Could you check a few things on this model? Use its own coordinates, in mm. A direction names the side the tool comes from. Coordinates: 2 decimals unless noted, no trailing zeros. Write each loop counter-clockwise with the first axis right and the second up, starting at its lowest first coordinate (ties: lowest second). Pieces come first, ordered by that corner, then holes.
Item 1: Which directions (+Z, -Z, +X, -X, +Y, -Y) give clear straight access to the entire face, cutting with the end or side of a thin tool? Please do faces 1 (the flat face through (-2, 2, -8.8)), 2 (the flat face through (-8.745, -7, 5)), 3 (the flat face through (-7.245, -5, 6)).
Item 2: I want a section at C-C on x = -13.5. Please give me the cut outline in (y, z), then the cut area to 3 significant figures.
Item 3: I want a section at B-B on y = -8. Please give me the cut outline in (x, z).
Item 4: If I drill on probe 1 along Z at (x, y) = (-4, -1.75); probe 2 along X at (y, z) = (-1.25, 0.5); probe 3 along Z at (x, y) = (-12.5, -1), over which ranges is the centre line in solid material (lowest first)?
Item 5: Thinking about a two-plate mould opening in X: for faces 4 (the flat face through (3.255, -3, 5)), 5 (the flat face through (1, 4, -19.7)), 6 (the flat face through (-8, -3, 8.8)), 7 (the cylindrical face through (1.54, 10.22, -5.87)), which applies, +X half, -X half, draft (parallel to the pull), parting line (faces both ways), or undercut?
Item 6: For P1, Ø1.6, axis at x = -3, y = -5.5, coming from the +Z side; P2, Ø1.5, axis at y = -3.5, z = 7, coming from the -X side; P3, Ø0.6, axis at y = 4, z = -20, coming from the -X side, each with a flat end and sliding along its axis, tell me the tip position at first contact or that it passes through.
Item 7: I want a section at A-A on z = 5. Please give me the cut outline in (x, y), then the cut area to 3 significant figures.
from build123d import *

# Parameters (mm, degrees)
ESQUISSE1_R             = 1.15
BOSS_EXTRU_1_DEPTH      = 1.8
BOSS_EXTRU_2_DEPTH      = 8
ENL_V_MAT_EXTRU_1_DEPTH = 7
ESQUISSE4_W             = 3.5
ESQUISSE4_H             = 0.873592076
ENL_V_MAT_EXTRU_2_DEPTH = 1
ESQUISSE5_W             = 1
ESQUISSE5_H             = 1
ENL_V_MAT_EXTRU_3_DEPTH = 11
ESQUISSE6_W             = 6.2
ESQUISSE6_H             = 3.3
ENL_V_MAT_EXTRU_4_DEPTH = 1
CHANFREIN1_SIZE         = 1
BOSS_EXTRU_3_DEPTH      = 4
ESQUISSE8_R             = 6.32
BOSS_EXTRU_4_DEPTH      = 4.8
CONG_1_R                = 1
ESQUISSE10_R            = 1.75
BOSS_EXTRU_5_DEPTH      = 1.6
CONG_2_R                = 1
ESQUISSE11_R            = 1.5
BOSS_EXTRU_6_DEPTH      = 10
ESQUISSE12_W            = 2.890262719
ESQUISSE12_H            = 1.095500593
ENL_V_MAT_EXTRU_7_DEPTH = 7
CHANFREIN2_SIZE         = 0.5
ESQUISSE13_W            = 1.2
ESQUISSE13_H            = 2.827300788
ENL_V_MAT_EXTRU_8_DEPTH = 0.7


with BuildPart() as part:
    # Esquisse1 → Boss.-Extru.1 (new body)
    with BuildSketch(Plane.XY):
        with BuildLine():
            Line((-12.744645331, 10.992907801), (-4.994645331, 10.992907801))
            ThreePointArc((-4.994645331, 10.992907801), (-2.744645331, 8.742907801), (-0.494645331, 10.992907801))
            Line((-0.494645331, 10.992907801), (7.255354669, 10.992907801))
            Line((7.255354669, 10.992907801), (7.255354669, 3.192907801))
            ThreePointArc((7.255354669, 3.192907801), (9.455354669, 0.992907801), (7.255354669, -1.207092199))
            Line((7.255354669, -1.207092199), (7.255354669, -9.007092199))
            Line((7.255354669, -9.007092199), (-0.494645331, -9.007092199))
            ThreePointArc((-0.494645331, -9.007092199), (-2.744645331, -6.757092199), (-4.994645331, -9.007092199))
            Line((-4.994645331, -9.007092199), (-12.744645331, -9.007092199))
            Line((-12.744645331, -9.007092199), (-12.744645331, -1.207092199))
            ThreePointArc((-12.744645331, -1.207092199), (-14.944645331, 0.992907801), (-12.744645331, 3.192907801))
            Line((-12.744645331, 3.192907801), (-12.744645331, 10.992907801))
        make_face()
        with Locations((-12.744645331, 0.992907801)):
            Circle(ESQUISSE1_R, mode=Mode.SUBTRACT)
        with Locations((7.255354669, 0.992907801)):
            Circle(ESQUISSE1_R, mode=Mode.SUBTRACT)
    extrude(amount=BOSS_EXTRU_1_DEPTH)

    # Esquisse2 → Boss.-Extru.2 (add)
    with BuildSketch(Plane.XY.offset(1.8)):
        Polygon((-8.744645331, -7.507092199), (3.255354669, -7.507092199), (3.255354669, -6.707092199), (2.255354669, -6.707092199), (2.255354669, -4.407092199), (3.255354669, -4.407092199), (3.255354669, -2.507092199), (-8.744645331, -2.507092199), (-8.744645331, -4.407092199), (-7.744645331, -4.407092199), (-7.744645331, -6.707092199), (-8.744645331, -6.707092199), align=None)
    extrude(amount=BOSS_EXTRU_2_DEPTH)

    # Esquisse3 → Enlèv. mat.-Extru.1 (cut)
    with BuildSketch(Plane.XY.offset(9.8)):
        Polygon((-6.444645331, -3.707092199), (0.955354669, -3.707092199), (0.955354669, -2.907092199), (1.755354669, -2.907092199), (1.755354669, -3.707092199), (1.755354669, -6.707092199), (-7.244645331, -6.707092199), (-7.244645331, -3.707092199), (-7.244645331, -2.907092199), (-6.444645331, -2.907092199), align=None)
    extrude(amount=-ENL_V_MAT_EXTRU_1_DEPTH, mode=Mode.SUBTRACT)

    # Esquisse4 → Enlèv. mat.-Extru.2 (cut)
    with BuildSketch(Plane(origin=(0, -2.507092199, 0), x_dir=(1, 0, 0), z_dir=(0, 1, 0))):
        Polygon((-8.744645331, -1.8), (3.255354669, -1.8), (3.255354669, -2.8), (0.455354669, -2.8), (0.455354669, -9.8), (-5.944645331, -9.8), (-5.944645331, -2.8), (-8.744645331, -2.8), align=None)
        with Locations((-2.744645331, -6.063203962)):
            Rectangle(ESQUISSE4_W, ESQUISSE4_H, mode=Mode.SUBTRACT)
    extrude(amount=-ENL_V_MAT_EXTRU_2_DEPTH, mode=Mode.SUBTRACT)

    # Esquisse5 → Enlèv. mat.-Extru.3 (cut)
    with BuildSketch(Plane(origin=(0, -2.507092199, 0), x_dir=(1, 0, 0), z_dir=(0, 1, 0))):
        with Locations((-8.244645331, -9.3)):
            Rectangle(ESQUISSE5_W, ESQUISSE5_H)
        with Locations((2.755354669, -9.3)):
            Rectangle(ESQUISSE5_W, ESQUISSE5_H)
    extrude(amount=-ENL_V_MAT_EXTRU_3_DEPTH, mode=Mode.SUBTRACT)

    # Esquisse6 → Enlèv. mat.-Extru.4 (cut)
    with BuildSketch(Plane(origin=(0, -3.507092199, 0), x_dir=(1, 0, 0), z_dir=(0, 1, 0))):
        with Locations((-2.744645331, -8.15)):
            Rectangle(ESQUISSE6_W, ESQUISSE6_H)
    extrude(amount=-ENL_V_MAT_EXTRU_4_DEPTH, mode=Mode.SUBTRACT)

    # Chanfrein1
    # the kernel refuses this chamfer: 1 mm, written as the material it takes off along each edge
    with BuildSketch(Plane(origin=(1.577037657, -2.507092199, 6.5), x_dir=(0, -0.9996219169112968, 0.027495876610586487), z_dir=(-1, 0, 0))) as chanfrein1_piece_1_section:
        Polygon((CHANFREIN1_SIZE * 0.999621916911, -CHANFREIN1_SIZE * 0.0274958766106), (-CHANFREIN1_SIZE * 0.0274958766106, -CHANFREIN1_SIZE * 0.999621916911), (0, 0), align=None)
    chanfrein1_piece_1 = extrude(amount=6.071682988, mode=Mode.PRIVATE)
    chanfrein1_piece_1 = split(chanfrein1_piece_1, bisect_by=Plane(origin=(0.455354669, -3.107092199, 6.3), z_dir=(-1, 0, 0)), keep=Keep.TOP, mode=Mode.PRIVATE)
    add(chanfrein1_piece_1, mode=Mode.SUBTRACT)

    # Esquisse7 → Boss.-Extru.3 (add)
    with BuildSketch(Plane(origin=(0, 0, 0), x_dir=(-1, 0, 0), z_dir=(0, 0, -1))):
        with BuildLine():
            Line((9.544645331, 10.292907801), (-0.715354669, 10.292907801))
            ThreePointArc((-0.715354669, 10.292907801), (-5.198411662, 8.435964794), (-7.055354669, 3.952907801))
            Line((-7.055354669, 3.952907801), (-7.055354669, 3.932907801))
            ThreePointArc((-7.055354669, 3.932907801), (-5.198411662, -0.550149191), (-0.715354669, -2.407092199))
            Line((-0.715354669, -2.407092199), (9.544645331, -2.407092199))
            Line((9.544645331, -2.407092199), (9.544645331, 10.292907801))
        make_face()
    extrude(amount=BOSS_EXTRU_3_DEPTH)

    # Esquisse8 → Boss.-Extru.4 (add)
    with BuildSketch(Plane(origin=(0, 0, -4), x_dir=(-1, 0, 0), z_dir=(0, 0, -1))):
        with Locations((-0.715354669, 3.952907801)):
            Circle(ESQUISSE8_R)
    extrude(amount=BOSS_EXTRU_4_DEPTH)

    # Congé1
    cong_1_edges = [part.edges().sort_by_distance(p)[0] for p in [
        (7.035354669, 3.952907801, -8.8),
    ]]
    fillet(cong_1_edges, radius=CONG_1_R)

    # Esquisse10 → Boss.-Extru.5 (add)
    with BuildSketch(Plane(origin=(0, 0, -8.8), x_dir=(-1, 0, 0), z_dir=(0, 0, -1))):
        with Locations((-0.715354669, 3.952907801)):
            Circle(ESQUISSE10_R)
    extrude(amount=BOSS_EXTRU_5_DEPTH)

    # Congé2
    cong_2_edges = [part.edges().sort_by_distance(p)[0] for p in [
        (2.465354669, 3.952907801, -8.8),
    ]]
    fillet(cong_2_edges, radius=CONG_2_R)

    # Esquisse11 → Boss.-Extru.6 (add)
    with BuildSketch(Plane(origin=(0, 0, -10.4), x_dir=(-1, 0, 0), z_dir=(0, 0, -1))):
        with Locations((-0.715354669, 3.952907801)):
            Circle(ESQUISSE11_R)
    extrude(amount=BOSS_EXTRU_6_DEPTH)

    # Esquisse12 → Enlèv. mat.-Extru.7 (cut)
    with BuildSketch(Plane(origin=(0, 0, -20.4), x_dir=(-1, 0, 0), z_dir=(0, 0, -1))):
        with Locations((-0.539081064, 5.300658098)):
            Rectangle(ESQUISSE12_W, ESQUISSE12_H)
    extrude(amount=-ENL_V_MAT_EXTRU_7_DEPTH, mode=Mode.SUBTRACT)

    # Chanfrein2
    chanfrein2_edges = [part.edges().sort_by_distance(p)[0] for p in [
        (1.131715912, 2.511851482, -20.4),
        (0.715354669, 4.752907801, -20.4),
    ]]
    chamfer(chanfrein2_edges, length=CHANFREIN2_SIZE)

    # Esquisse13 → Enlèv. mat.-Extru.8 (cut)
    with BuildSketch(Plane(origin=(0, 0, -20.4), x_dir=(-1, 0, 0), z_dir=(0, 0, -1))):
        with Locations((-0.715354669, 3.515442174)):
            Rectangle(ESQUISSE13_W, ESQUISSE13_H)
    extrude(amount=-ENL_V_MAT_EXTRU_8_DEPTH, mode=Mode.SUBTRACT)


solid = part.part
Response values:
1. face 1: -Z
1. face 2: +Z, -X, +Y, -Y
1. face 3: +Z
2. outline: (-1.07, 0) - (0.13, 0) - (0.13, 1.8) - (-1.07, 1.8) - close; (1.86, 0) - (3.06, 0) - (3.06, 1.8) - (1.86, 1.8) - close
2. area: 4.32 mm2
3. outline: (-12.74, 0) - (-4.76, 0) - (-4.76, 1.8) - (-12.74, 1.8) - close; (-0.73, 0) - (7.26, 0) - (7.26, 1.8) - (-0.73, 1.8) - close
4. probe 1: z = -4 to 1.8
4. probe 2: x = -12.74 to 7.26
4. probe 3: z = 0 to 1.8
5. face 4: +X half
5. face 5: undercut
5. face 6: draft
5. face 7: parting line
6. P1: stops at z = 2.8
6. P2: stops at x = -8.74
6. P3: stops at x = -0.78
7. outline: (-8.74, -7.51) - (3.26, -7.51) - (3.26, -6.71) - (2.26, -6.71) - (2.26, -4.41) - (3.26, -4.41) - (3.26, -2.51) - (0.46, -2.51) - (0.46, -3.51) - (-5.94, -3.51) - (-5.94, -2.51) - (-8.74, -2.51) - (-8.74, -4.41) - (-7.74, -4.41) - (-7.74, -6.71) - (-8.74, -6.71) - close; hole (-7.24, -6.71) - (1.76, -6.71) - (1.76, -2.91) - (0.96, -2.91) - (0.96, -3.71) - (-6.44, -3.71) - (-6.44, -2.91) - (-7.24, -2.91) - close
7. area: 20.7 mm2
